The model under review builds one solid part; all positions refer to its coordinate system, in mm. Face numbers are marked on the shaded views. A direction names the side the tool comes from. Coordinates: 2 decimals unless noted, no trailing zeros. Order: outer loops, then holes, each group sorted by start corner. A loop starts at its lowest first (then second) coordinate and runs counter-clockwise, first axis right, second up. Notation, with made-up numbers: (85, -24.75) -> (120, -24.75) arc R36 ccw to (120, 10.25) -> close; hole circle Ø3 at (65, 31). An arc over 180 degrees is marked (long way). Use one line per item in the form item = value.
Solid Edge part; units mm, degrees
sketch "Sketch1" plane through (0, 0, 0) normal (0, -1, 0) x (1, 0, 0)
  line L0 (8, 53) -> (8, 8)
  line L1 (8, 8) -> (58, 8)
  line L2 (58, 8) -> (58, 0)
  line L3 (58, 0) -> (0, 0)
  line L4 (0, 0) -> (0, 53)
  line L5 (0, 53) -> (8, 53)
extrude "Extrusionsausprägung_16" add sketch "Sketch1" against normal blind 35
sketch "Sketch2" plane through (39, 25, 8) normal (0, 0, 1) x (-1, 0, 0)
  circle A0 centre (26, 20) radius 2.25
  circle A1 centre (-14, 20) radius 2.25
  circle A2 centre (-14, -5) radius 2.25
  circle A3 centre (26, -5) radius 2.25
extrude "Extrusionsausschnitt_23" cut sketch "Sketch2" against normal blind 79.6572
extrude "Cutout1" [suppressed]
sketch "Sketch3" plane through (8, 17.5, 29) normal (1, 0, 0) x (0, 0, 1)
  line L0 (19, 12.5) -> (-16, 12.5)
  line L1 (-16, 12.5) -> (-16, 6.2)
  line L2 (-16, 6.2) -> (19, 6.2)
  line L3 (19, 6.2) -> (19, 12.5)
extrude "Extrusionsausschnitt_25" cut sketch "Sketch3" against normal blind 90.2255
fillet "Verrundung_15" radius 3.15 4 edges at (4, 11.3, 13) (4, 5, 13) (4, 5, 48) (4, 11.3, 48)
mirror "Mirror1" about plane through (29, 17.5, 25) normal (0, -1, 0) of "Extrusionsausschnitt_25", "Verrundung_15"
sketch "Sketch4" plane through (4, 17.5, 53) normal (0, 0, 1) x (-1, 0, 0)
  line L0 (2, 17.5) -> (2, 4)
  line L1 (2, 4) -> (4, 4)
  line L2 (4, 4) -> (4, 17.5)
  line L3 (4, 17.5) -> (2, 17.5)
extrude "Extrusionsausschnitt_26" cut sketch "Sketch4" against normal blind 65.9073
mirror "Mirror2" about plane through (29, 17.5, 25) normal (0, -1, 0) of "Extrusionsausschnitt_26"
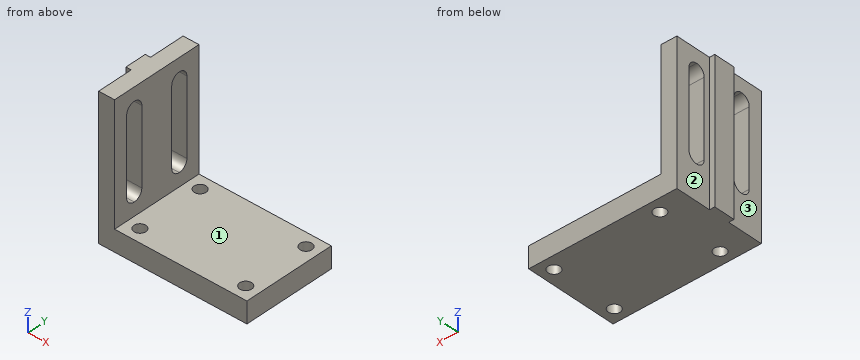
Item 1: We need section C-C (z = 32). Write out the cut boundary in (x, y), plus the area to 3 significant figures.
Results found:
outline = (0, 13.5) -> (2, 13.5) -> (2, 11.3) -> (8, 11.3) -> (8, 23.7) -> (2, 23.7) -> (2, 21.5) -> (0, 21.5) -> close; (2, 0) -> (8, 0) -> (8, 5) -> (2, 5) -> close; (2, 30) -> (8, 30) -> (8, 35) -> (2, 35) -> close
area = 150 mm²
Item 2: Clearance check with flat-ended pins moving along their axes: pin 1 (1 mm diameter, centred on x = 17.5, y = 25, fed in from -Z); pin 2 (6 mm diameter, centred on x = 13, y = 5, fed in from +Z); pin 3 (7 mm diameter, centred on y = 31, z = 29, fed in from -X); pin 4 (1.6 mm diameter, centred on x = 1, z = 19, fed in from +Y). State where each tip first meets the part, or that it passes through.
Results found:
pin_1 = 0
pin_2 = 8
pin_3 = 2
pin_4 = 21.5
Item 3: We need section B-B (z = 7). Write out the cut boundary in (x, y).
Results found:
outline = (0, 13.5) -> (2, 13.5) -> (2, 0) -> (58, 0) -> (58, 35) -> (2, 35) -> (2, 21.5) -> (0, 21.5) -> close; hole circle Ø4.5 at (13, 5); hole circle Ø4.5 at (13, 30); hole circle Ø4.5 at (53, 5); hole circle Ø4.5 at (53, 30)
Item 4: To check wall thickness, follow L1, parallel to Y at x = 13, z = 3; L2, parallel to X at y = 5, z = 5.75; L3, parallel to Z at x = 39.5, y = 18. State the ranges of each line that lie inside material, in increasing order. Write a range as from..to.
Results found:
L1 = 0..2.75, 7.25..27.75, 32.25..35
L2 = 2..10.75, 15.25..50.75, 55.25..58
L3 = 0..8
Item 5: Tool access review of the marked faces 1, 2 and 3: name each direction out of +Z, -Z, +X, -X, +Y, -Y from which nothing blocks a thin tool from reaching the whole face with its end or side.
Results found:
face_1 = +Z, +X, +Y, -Y
face_2 = +Z, -Z, -X, +Y
face_3 = +Z, -Z, -X, -Y
Item 6: We need section A-A (x = 13). Write out the cut boundary in (y, z).
Results found:
outline = (0, 0) -> (2.75, 0) -> (2.75, 8) -> (0, 8) -> close; (7.25, 0) -> (27.75, 0) -> (27.75, 8) -> (7.25, 8) -> close; (32.25, 0) -> (35, 0) -> (35, 8) -> (32.25, 8) -> close
Item 7: We need section D-D (y = 12). Write out the cut boundary in (x, z), plus the area to 3 significant figures.
Results found:
outline = (2, 0) -> (58, 0) -> (58, 8) -> (8, 8) -> (8, 53) -> (2, 53) -> close
area = 718 mm²
